Geometry check sheet. Reference: the model listing, model coordinates, mm. Face numbers are marked on the shaded views. A direction names the side the tool comes from. Give positions to 0.01 mm unless a question says otherwise; leave off trailing zeros. Loops run counter-clockwise (first coordinate to the right, second up) from the corner with the lowest first, then second, coordinate; pieces in that order, holes last.
1. Cross-section at B-B, the plane z = 14.5. Record the cut outline in (x, y) (3 decimals), plus the area to 3 significant figures.
2. Cross-section at A-A, the plane y = 23. Record the cut outline in (x, z), plus the area to 3 significant figures.
3. Tool access check on the marked faces 1, 2 and 3. Record the directions out of +Z, -Z, +X, -X, +Y, -Y that give a thin tool (end or side, any length) a straight path to the whole face; none if there is none.
4. Material ranges on L1, parallel to Y at x = 4.5, z = -12.7 (3 decimals); L2, parallel to Y at x = 24, z = 0 (3 decimals); L3, parallel to X at y = 23, z = -6, recorded low to high.
5. Release check for a two-part mould opening along Z. For the marked faces 4, 5 and 6 record: +Z half, -Z half, draft (parallel to the pull), parting line (faces both ways), or undercut.
6. Go/stop test with flat-tipped pins: pin 1 Ø1.5 at (y, z) = (-13, 1) entering from +X; pin 2 Ø6 at (x, z) = (12, 5.5) entering from -Y (3 decimals); pin 3 Ø1.3 at (x, y) = (13.5, 30) entering from -Z; pin 4 Ø20.5 at (y, z) = (30.5, 3.5) entering from -X. Record where each tip stops, or that it passes through.
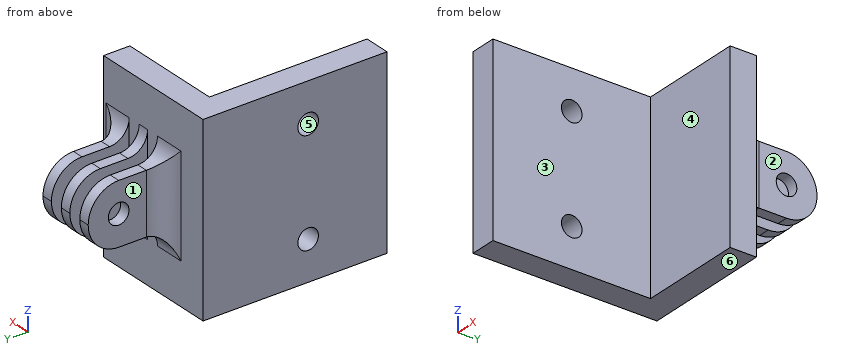
from build123d import *

# Parameters (mm, degrees)
SKETCH1_W           = 44.45
SKETCH1_H           = 44.45
SKETCH1_R           = 2.4892
BOSS_EXTRUDE1_DEPTH = 6.35
SKETCH2_W           = 44.45
SKETCH2_H           = 6.35
BOSS_EXTRUDE2_DEPTH = 25.4
SKETCH3_W           = 2.6924
SKETCH3_H           = 14.732
BOSS_EXTRUDE3_DEPTH = 18.796
FILLET3_R           = 7.366
CUT_EXTRUDE1_REACH  = 52.727
SKETCH4_R           = 2.4892
FILLET4_R           = 4.7625


with BuildPart() as part:
    # Sketch1 → Boss-Extrude1 (new body)
    with BuildSketch(Plane(origin=(0, 0, 0), x_dir=(0, 0, -1), z_dir=(1, 0, 0))):
        Rectangle(SKETCH1_W, SKETCH1_H)
        with Locations((-12.7, -3.175)):
            Circle(SKETCH1_R, mode=Mode.SUBTRACT)
        with Locations((12.7, -3.175)):
            Circle(SKETCH1_R, mode=Mode.SUBTRACT)
    extrude(amount=BOSS_EXTRUDE1_DEPTH)

    # Sketch2 → Boss-Extrude2 (add)
    with BuildSketch(Plane(origin=(6.35, 0, 0), x_dir=(0, 0, -1), z_dir=(1, 0, 0))):
        with Locations((0, 19.05)):
            Rectangle(SKETCH2_W, SKETCH2_H)
    extrude(amount=BOSS_EXTRUDE2_DEPTH)

    # Sketch3 → Boss-Extrude3 (add)
    with BuildSketch(Plane(origin=(0, 22.225, 0), x_dir=(1, 0, 0), z_dir=(0, 1, 0))):
        with Locations((13.1826, 0)):
            Rectangle(SKETCH3_W, SKETCH3_H)
        with Locations((19.05, 0)):
            Rectangle(SKETCH3_W, SKETCH3_H)
        with Locations((24.9174, 0)):
            Rectangle(SKETCH3_W, SKETCH3_H)
    extrude(amount=BOSS_EXTRUDE3_DEPTH)

    # Fillet3
    fillet3_edges = [part.edges().sort_by_distance(p)[0] for p in [
        (19.05, 41.021, -7.366),
        (13.1826, 41.021, -7.366),
        (24.9174, 41.021, 7.366),
        (19.05, 41.021, 7.366),
        (13.1826, 41.021, 7.366),
        (24.9174, 41.021, -7.366),
    ]]
    fillet(fillet3_edges, radius=FILLET3_R - 0.0001)  # a hair under: the kernel refuses the full size

    # Cut-Extrude1: up to this face of the body (flat: up to its plane)
    cut_extrude1_end = Plane(part.part.faces().sort_by_distance((26.2636, 30.911144625, 0))[0])
    # Sketch4 → Cut-Extrude1 (cut, up to the picked face)
    with BuildSketch(Plane.ZY.offset(-11.8364), mode=Mode.PRIVATE) as cut_extrude1_sk1:
        with Locations((0, 33.655)):
            Circle(SKETCH4_R)
    cut_extrude1_tool1 = split(extrude(cut_extrude1_sk1.sketch, amount=-CUT_EXTRUDE1_REACH, mode=Mode.PRIVATE), bisect_by=cut_extrude1_end, keep=Keep.BOTH, mode=Mode.PRIVATE)
    add(cut_extrude1_tool1.solids().sort_by(Axis((11.8364, 33.655, 0), (1, 0, 0)))[0], mode=Mode.SUBTRACT)

    # Fillet4
    fillet4_edges = [part.edges().sort_by_distance(p)[0] for p in [
        (13.1826, 22.225, -7.366),
        (11.8364, 22.225, 0),
        (13.1826, 22.225, 7.366),
        (19.05, 22.225, -7.366),
        (19.05, 22.225, 7.366),
        (24.9174, 22.225, -7.366),
        (24.9174, 22.225, 7.366),
        (26.2636, 22.225, 0),
    ]]
    fillet(fillet4_edges, radius=FILLET4_R)


solid = part.part
Result:
1. outline: (0, -22.225) - (6.35, -22.225) - (6.35, -4.894) - (0, -4.894) - close; (0, -1.456) - (6.35, -1.456) - (6.35, 15.875) - (31.75, 15.875) - (31.75, 22.225) - (0, 22.225) - close
1. area: 422 mm2
2. outline: (9.68, -9.52) - (14.53, -9.52) - (14.53, 9.52) - (9.68, 9.52) - close; (17.7, -9.52) - (20.4, -9.52) - (20.4, 9.52) - (17.7, 9.52) - close; (23.57, -9.52) - (28.42, -9.52) - (28.42, 9.52) - (23.57, 9.52) - close
2. area: 236 mm2
3. face 1: +Z, -Z, -X, +Y
3. face 2: +Z, -Z, +X, +Y
3. face 3: +Z, -Z, +X, -Y
4. L1: y = -22.225 to -5.664, -0.686 to 22.225
4. L2: y = 15.875 to 31.166, 36.144 to 41.021
4. L3: x = 9.68 to 14.53, 17.7 to 20.4, 23.57 to 28.42
5. face 4: draft
5. face 5: undercut
5. face 6: -Z half
6. pin 1: stops at x = 6.35
6. pin 2: stops at y = 15.875
6. pin 3: stops at z = -7.37
6. pin 4: stops at x = 0
